Source: CAD feature listing. Evaluate the final solid. Frame: model axes, mm. Round coordinates to 2 decimals unless told otherwise and drop trailing zeros. Write each loop counter-clockwise with the first axis right and the second up, starting at its lowest first coordinate (ties: lowest second). Pieces come first, ordered by that corner, then holes. Notation, with made-up numbers: (22.5, 63) -> (75.5, 63) arc R35 ccw to (75.5, 97) -> close; hole circle Ø1 at (-39, -32.75). An arc over 180 degrees is marked (long way). Put each result on its own line as item: value.
Autodesk Inventor part; units mm, degrees
ref_plane "YZ Plane" through (0, 0, 0) normal (1, 0, 0) x (0, 1, 0)
ref_plane "XZ Plane" through (0, 0, 0) normal (0, 1, 0) x (-1, 0, 0)
ref_plane "XY Plane" through (0, 0, 0) normal (0, 0, 1) x (1, 0, 0)
sketch "Boceto1" plane through (0, 0, 0) normal (0, 1, 0) x (-1, 0, 0)
  line L0 (0, 0) -> (-13, 0)
  line L1 (-13, 0) -> (-13, -8)
  line L2 (-13, -8) -> (0, -8)
  line L3 (0, -8) -> (0, 0)
  circle A0 centre (-11.9, -4) radius 1
  dimension "d0" = 13
  dimension "d1" = 8
  dimension "d2" = 2
  dimension "d3" = 1.1
  dimension "d4" = 4
  dimension "d5" = 4
extrude "Extrusión1" add sketch "Boceto1" along normal blind 2
equation "\"Radio_pliegue\" = Grosor"
equation "\"Anchura_desahogo_plegado\" = Grosor"
equation "\"Profundidad_desahogo_plegado\" = 0.5 * Grosor"
equation "\"Tamaño_destalonado\" = 4 * Grosor"
equation "\"Remanente_mínimo\" = 2 * Grosor"
equation "\"Radiodetransición\" = Radio_pliegue"
equation "\"Tamaño_de_radio_de_Jacobi\" = Radio_pliegue"
equation "\"TamañoSeparación\" = Grosor"
properties part number "SensorDeLinea"
Q1. Cut plane C-C on z = -3.25. Output: boundary loops of the cut face in (x, y), and give its area (3 significant figures).
Ans:
outline: (0, 0) -> (11.24, 0) -> (11.24, 2) -> (0, 2) -> close; (12.56, 0) -> (13, 0) -> (13, 2) -> (12.56, 2) -> close
area: 23.4 mm^2
Q2. Cut plane B-B on y = 1.7. Output: boundary loops of the cut face in (x, z), and give its area (3 significant figures).
Ans:
outline: (0, -8) -> (13, -8) -> (13, 0) -> (0, 0) -> close; hole circle Ø2 at (11.9, -4)
area: 101 mm^2
Q3. Draft query along Y for faces 1 (the flat face through (7, 2, -4)), 2 (the flat face through (0, 1, -4)), 3 (the flat face through (7, 0, -4)). Return one class per face: +Y half, -Y half, draft (parallel to the pull), parting line (faces both ways), or undercut.
Ans:
face 1: +Y half
face 2: draft
face 3: -Y half
Q4. Pin query (flat end, axial travel): pin 1 (3 mm diameter, centred on x = 11.9, z = -4, fed in from +Y). Return the tip coordinate at first contact, or that it passes through.
Ans:
pin 1: stops at y = 2
Q5. Cut plane A-A on x = 11.9. Output: boundary loops of the cut face in (y, z).
Ans:
outline: (0, -8) -> (2, -8) -> (2, -5) -> (0, -5) -> close; (0, -3) -> (2, -3) -> (2, 0) -> (0, 0) -> close
Q6. Material intervals for line 1 (Z direction, x = 11.9, y = 0.55); line 2 (Z direction, x = 11.5, y = 1.75), sorted ascending. Write a range as [from, to].
Ans:
line 1: z = [-8, -5], [-3, 0]
line 2: z = [-8, -4.92], [-3.08, 0]
